```python
from build123d import *

# Parameters (mm, degrees)
SKETCH1_W                       = 165.076666628
SKETCH1_H                       = 208.28
BOSS_EXTRUDE1_DEPTH             = 89.481016872
SKETCH3_W                       = 161.266666628
SKETCH3_H                       = 208.28
CUT_EXTRUDE1_DEPTH              = 87.576016872
F_6_CLEARANCE_HOLE1_AT_2_COUNT  = 2
F_6_CLEARANCE_HOLE1_AT_2_PITCH  = 70.431016872
F_6_CLEARANCE_HOLE1_AT_3_COUNT  = 2
F_6_CLEARANCE_HOLE1_AT_3_PITCH  = 201.912161688
F_6_CLEARANCE_HOLE1_AT_4_COUNT  = 2
F_6_CLEARANCE_HOLE1_AT_4_PITCH  = 189.23
F_6_CLEARANCE_HOLE2_D           = 4.3053
F_6_CLEARANCE_HOLE2_DEPTH       = 6.858
F_6_CLEARANCE_HOLE2_CSINK_D     = 6.6548
F_6_CLEARANCE_HOLE2_CSINK_ANGLE = 90
F_6_CLEARANCE_HOLE2_TIP         = 1.293442612
CUT_EXTRUDE2_REACH              = 162.202
SKETCH8_R                       = 45.72
CUT_EXTRUDE3_REACH              = 162.202
SKETCH9_R                       = 6
SKETCH9_W                       = 101.6
SKETCH9_H                       = 25.4
CUT_EXTRUDE4_DEPTH              = 0.9525
CUT_EXTRUDE6_REACH              = 162.202
SKETCH13_R                      = 6.35
CUT_EXTRUDE7_DEPTH              = 1
CHAMFER1_SIZE                   = 1


# Read off the part's stored shape, not the designer's step: M2 Clearance Hole1
with BuildPart() as part:
    # Sketch1 → Boss-Extrude1 (new body)
    with BuildSketch(Plane(origin=(0, 0, 0), x_dir=(0, 0, -1), z_dir=(1, 0, 0))):
        Rectangle(SKETCH1_W, SKETCH1_H)
    extrude(amount=BOSS_EXTRUDE1_DEPTH)

    # Sketch3 → Cut-Extrude1 (cut)
    with BuildSketch(Plane.ZY):
        Rectangle(SKETCH3_W, SKETCH3_H)
    extrude(amount=-CUT_EXTRUDE1_DEPTH, mode=Mode.SUBTRACT)

    # Sketch5 → #6 Clearance Hole1 (revolve, cut)
    with BuildSketch(Plane(origin=(9.525, -94.615, -82.538333314), x_dir=(0, 1, 0), z_dir=(1, 0, 0))):
        Polygon((0, 0), (0, 1.905), (2.15265, 1.905), (2.15265, 1.17475), (3.3274, 0), align=None)
    f_6_clearance_hole1 = revolve(axis=Axis((9.525, -94.615, -88.888333314), (0, 0, 1)), mode=Mode.SUBTRACT)

    # #6 Clearance Hole1 at 2: #6 Clearance Hole1 ×2
    with Locations(*[(i * F_6_CLEARANCE_HOLE1_AT_2_PITCH, 0, 0) for i in range(1, F_6_CLEARANCE_HOLE1_AT_2_COUNT)]):
        add(f_6_clearance_hole1, mode=Mode.SUBTRACT)

    # #6 Clearance Hole1 at 3: #6 Clearance Hole1 ×2
    with Locations(*[Vector(0.34882008237197215, 0.9371897087217778, 0) * (i * F_6_CLEARANCE_HOLE1_AT_3_PITCH) for i in range(1, F_6_CLEARANCE_HOLE1_AT_3_COUNT)]):
        add(f_6_clearance_hole1, mode=Mode.SUBTRACT)

    # #6 Clearance Hole1 at 4: #6 Clearance Hole1 ×2
    with Locations(*[(0, i * F_6_CLEARANCE_HOLE1_AT_4_PITCH, 0) for i in range(1, F_6_CLEARANCE_HOLE1_AT_4_COUNT)]):
        add(f_6_clearance_hole1, mode=Mode.SUBTRACT)

    # #6 Clearance Hole2
    with Locations(Plane.XY.offset(82.538333314)):
        with Locations((9.525, 94.615), (79.956016872, 94.615), (79.956016872, -94.615), (9.525, -94.615)):
            CounterSinkHole(F_6_CLEARANCE_HOLE2_D / 2, F_6_CLEARANCE_HOLE2_CSINK_D / 2, depth=F_6_CLEARANCE_HOLE2_DEPTH, counter_sink_angle=F_6_CLEARANCE_HOLE2_CSINK_ANGLE)
            with Locations((0, 0, -(F_6_CLEARANCE_HOLE2_DEPTH + F_6_CLEARANCE_HOLE2_TIP / 2))):  # 118° drill point
                Cone(0, F_6_CLEARANCE_HOLE2_D / 2, F_6_CLEARANCE_HOLE2_TIP, mode=Mode.SUBTRACT)

    # Sketch8 → Cut-Extrude2 (cut, up to next)
    with BuildSketch(Plane(origin=(89.481016872, 0, 0), x_dir=(0, 0, -1), z_dir=(1, 0, 0)), mode=Mode.PRIVATE) as cut_extrude2_sk1:
        with Locations((15.193333225, 51.676666667)):
            Circle(SKETCH8_R)
    cut_extrude2_tool1 = extrude(cut_extrude2_sk1.sketch, amount=-CUT_EXTRUDE2_REACH, mode=Mode.PRIVATE) & part.part
    add(cut_extrude2_tool1.solids().sort_by_distance((89.481017, 51.676667, -15.193333))[0], mode=Mode.SUBTRACT)

    # Sketch9 → Cut-Extrude3 (cut, up to next)
    with BuildSketch(Plane(origin=(89.481016872, 0, 0), x_dir=(0, 0, -1), z_dir=(1, 0, 0)), mode=Mode.PRIVATE) as cut_extrude3_sk1:
        with Locations((55.233333314, -52.07)):
            Circle(SKETCH9_R)
    cut_extrude3_tool1 = extrude(cut_extrude3_sk1.sketch, amount=-CUT_EXTRUDE3_REACH, mode=Mode.PRIVATE) & part.part
    # Sketch9 → Cut-Extrude3 (cut, up to next)
    with BuildSketch(Plane(origin=(89.481016872, 0, 0), x_dir=(0, 0, -1), z_dir=(1, 0, 0)), mode=Mode.PRIVATE) as cut_extrude3_sk2:
        with Locations((-11.418333314, -33.02)):
            Rectangle(SKETCH9_W, SKETCH9_H)
    cut_extrude3_tool2 = extrude(cut_extrude3_sk2.sketch, amount=-CUT_EXTRUDE3_REACH, mode=Mode.PRIVATE) & part.part
    # Sketch9 → Cut-Extrude3 (cut, up to next)
    with BuildSketch(Plane(origin=(89.481016872, 0, 0), x_dir=(0, 0, -1), z_dir=(1, 0, 0)), mode=Mode.PRIVATE) as cut_extrude3_sk3:
        with Locations((-11.418333314, -71.12)):
            Rectangle(SKETCH9_W, SKETCH9_H)
    cut_extrude3_tool3 = extrude(cut_extrude3_sk3.sketch, amount=-CUT_EXTRUDE3_REACH, mode=Mode.PRIVATE) & part.part
    add(cut_extrude3_tool1.solids().sort_by_distance((89.481017, -52.07, -55.233333))[0], mode=Mode.SUBTRACT)
    add(cut_extrude3_tool2.solids().sort_by_distance((89.481017, -33.02, 11.418333))[0], mode=Mode.SUBTRACT)
    add(cut_extrude3_tool3.solids().sort_by_distance((89.481017, -71.12, 11.418333))[0], mode=Mode.SUBTRACT)

    # M2 Clearance Hole1 outline → M2 Clearance Hole1 (revolve, cut)
    with BuildSketch(Plane(origin=(0, -33.02, 65.393333314), x_dir=(0, 1, 0), z_dir=(0, 0, -1))):
        Polygon((0, 87.576016872), (1.3, 87.576016872), (1.3, 88.881016872), (1.9, 89.481016872), (0, 89.481016872), align=None)
    revolve(axis=Axis((0, -33.02, 65.393333314), (1, 0, 0)), mode=Mode.SUBTRACT)

    # M2 Clearance Hole1 2 outline → M2 Clearance Hole1 2 (revolve, cut)
    with BuildSketch(Plane(origin=(0, -33.02, -42.556666686), x_dir=(0, 1, 0), z_dir=(0, 0, -1))):
        Polygon((0, 87.576016872), (1.3, 87.576016872), (1.3, 88.881016872), (1.9, 89.481016872), (0, 89.481016872), align=None)
    revolve(axis=Axis((0, -33.02, -42.556666686), (1, 0, 0)), mode=Mode.SUBTRACT)

    # M2 Clearance Hole1 3 outline → M2 Clearance Hole1 3 (revolve, cut)
    with BuildSketch(Plane(origin=(0, -71.12, -42.556666686), x_dir=(0, 1, 0), z_dir=(0, 0, -1))):
        Polygon((0, 87.576016872), (1.3, 87.576016872), (1.3, 88.881016872), (1.9, 89.481016872), (0, 89.481016872), align=None)
    revolve(axis=Axis((0, -71.12, -42.556666686), (1, 0, 0)), mode=Mode.SUBTRACT)

    # M2 Clearance Hole1 4 outline → M2 Clearance Hole1 4 (revolve, cut)
    with BuildSketch(Plane(origin=(0, -71.12, 65.393333314), x_dir=(0, 1, 0), z_dir=(0, 0, -1))):
        Polygon((0, 87.576016872), (1.3, 87.576016872), (1.3, 88.881016872), (1.9, 89.481016872), (0, 89.481016872), align=None)
    revolve(axis=Axis((0, -71.12, 65.393333314), (1, 0, 0)), mode=Mode.SUBTRACT)

    # Sketch12 → Cut-Extrude4 (cut)
    with BuildSketch(Plane.ZY.offset(-87.576016872)):
        with BuildLine():
            Line((-39.381666686, -17.78), (62.218333314, -17.78))
            Line((62.218333314, -17.78), (66.304587615, -24.952694807))
            ThreePointArc((66.304587615, -24.952694807), (68.441333314, -33.02), (66.304587615, -41.087305193))
            Line((66.304587615, -41.087305193), (62.218333314, -48.26))
            Line((62.218333314, -48.26), (-39.381666686, -48.26))
            Line((-39.381666686, -48.26), (-43.467920986, -41.087305193))
            ThreePointArc((-43.467920986, -41.087305193), (-45.604666686, -33.02), (-43.467920986, -24.952694807))
            Line((-43.467920986, -24.952694807), (-39.381666686, -17.78))
        make_face()
        with BuildLine():
            Line((-43.467920986, -79.187305193), (-39.381666686, -86.36))
            Line((-39.381666686, -86.36), (62.218333314, -86.36))
            Line((62.218333314, -86.36), (66.304587615, -79.187305193))
            ThreePointArc((66.304587615, -79.187305193), (68.441333314, -71.12), (66.304587615, -63.052694807))
            Line((66.304587615, -63.052694807), (62.218333314, -55.88))
            Line((62.218333314, -55.88), (-39.381666686, -55.88))
            Line((-39.381666686, -55.88), (-43.467920986, -63.052694807))
            ThreePointArc((-43.467920986, -63.052694807), (-45.604666686, -71.12), (-43.467920986, -79.187305193))
        make_face()
    extrude(amount=-CUT_EXTRUDE4_DEPTH, mode=Mode.SUBTRACT)

    # Lettering Outline → Cut-Extrude6 (cut, up to next)
    with BuildSketch(Plane(origin=(89.481016872, 0, 0), x_dir=(0, 0, -1), z_dir=(1, 0, 0)), mode=Mode.PRIVATE) as cut_extrude6_sk1:
        Polygon((-62.218333314, 78.77), (-62.218333314, 75.383333333), (-52.058333314, 75.383333333), (-52.058333314, 71.996666667), (-62.218333314, 71.996666667), (-62.218333314, 61.836666667), (-55.444999981, 61.836666667), (-55.444999981, 68.61), (-48.671666648, 61.836666667), (-45.284999981, 61.836666667), (-45.284999981, 65.223333333), (-48.671666648, 68.61), (-45.284999981, 68.61), (-45.284999981, 78.77), align=None)
    cut_extrude6_tool1 = extrude(cut_extrude6_sk1.sketch, amount=-CUT_EXTRUDE6_REACH, mode=Mode.PRIVATE) & part.part
    # Lettering Outline → Cut-Extrude6 (cut, up to next)
    with BuildSketch(Plane(origin=(89.481016872, 0, 0), x_dir=(0, 0, -1), z_dir=(1, 0, 0)), mode=Mode.PRIVATE) as cut_extrude6_sk2:
        Polygon((-62.218333314, 80.463333333), (-62.218333314, 90.623333333), (-52.058333314, 90.623333333), (-52.058333314, 94.01), (-62.218333314, 94.01), (-62.218333314, 97.396666667), (-45.284999981, 97.396666667), (-45.284999981, 80.463333333), (-52.058333314, 80.463333333), (-52.058333314, 87.236666667), (-55.444999981, 87.236666667), (-55.444999981, 80.463333333), align=None)
    cut_extrude6_tool2 = extrude(cut_extrude6_sk2.sketch, amount=-CUT_EXTRUDE6_REACH, mode=Mode.PRIVATE) & part.part
    # Lettering Outline → Cut-Extrude6 (cut, up to next)
    with BuildSketch(Plane(origin=(89.481016872, 0, 0), x_dir=(0, 0, -1), z_dir=(1, 0, 0)), mode=Mode.PRIVATE) as cut_extrude6_sk3:
        Polygon((-62.218333314, 24.583333333), (-62.218333314, 34.743333333), (-52.058333314, 34.743333333), (-52.058333314, 38.13), (-62.218333314, 38.13), (-62.218333314, 41.516666667), (-45.284999981, 41.516666667), (-45.284999981, 24.583333333), (-52.058333314, 24.583333333), (-52.058333314, 31.356666667), (-55.444999981, 31.356666667), (-55.444999981, 24.583333333), align=None)
    cut_extrude6_tool3 = extrude(cut_extrude6_sk3.sketch, amount=-CUT_EXTRUDE6_REACH, mode=Mode.PRIVATE) & part.part
    # Lettering Outline → Cut-Extrude6 (cut, up to next)
    with BuildSketch(Plane(origin=(89.481016872, 0, 0), x_dir=(0, 0, -1), z_dir=(1, 0, 0)), mode=Mode.PRIVATE) as cut_extrude6_sk4:
        Polygon((-62.218333314, 5.956666667), (-62.218333314, 22.89), (-55.444999981, 22.89), (-55.444999981, 19.503333333), (-52.058333314, 16.116666667), (-52.058333314, 22.89), (-45.284999981, 22.89), (-45.284999981, 5.956666667), (-52.058333314, 5.956666667), (-52.058333314, 9.343333333), (-55.444999981, 12.73), (-55.444999981, 5.956666667), align=None)
    cut_extrude6_tool4 = extrude(cut_extrude6_sk4.sketch, amount=-CUT_EXTRUDE6_REACH, mode=Mode.PRIVATE) & part.part
    # Lettering Outline → Cut-Extrude6 (cut, up to next)
    with BuildSketch(Plane(origin=(89.481016872, 0, 0), x_dir=(0, 0, -1), z_dir=(1, 0, 0)), mode=Mode.PRIVATE) as cut_extrude6_sk5:
        Polygon((-62.218333314, 43.21), (-58.831666648, 43.21), (-58.831666648, 49.983333333), (-55.444999981, 49.983333333), (-55.444999981, 43.21), (-52.058333314, 43.21), (-52.058333314, 49.983333333), (-48.671666648, 49.983333333), (-48.671666648, 43.21), (-45.284999981, 43.21), (-45.284999981, 60.143333333), (-52.058333314, 60.143333333), (-52.058333314, 56.756666667), (-55.444999981, 56.756666667), (-55.444999981, 60.143333333), (-62.218333314, 60.143333333), align=None)
    cut_extrude6_tool5 = extrude(cut_extrude6_sk5.sketch, amount=-CUT_EXTRUDE6_REACH, mode=Mode.PRIVATE) & part.part
    add(cut_extrude6_tool1.solids().sort_by_distance((89.481017, 70.491481, 53.476681))[0], mode=Mode.SUBTRACT)
    add(cut_extrude6_tool2.solids().sort_by_distance((89.481017, 88.93, 53.243667))[0], mode=Mode.SUBTRACT)
    add(cut_extrude6_tool3.solids().sort_by_distance((89.481017, 33.05, 53.243667))[0], mode=Mode.SUBTRACT)
    add(cut_extrude6_tool4.solids().sort_by_distance((89.481017, 14.423333, 53.751667))[0], mode=Mode.SUBTRACT)
    add(cut_extrude6_tool5.solids().sort_by_distance((89.481017, 52.354, 53.751667))[0], mode=Mode.SUBTRACT)

    # Sketch13 → Cut-Extrude7 (cut)
    with BuildSketch(Plane.XY.offset(-80.633333314)):
        with Locations((79.956016872, 94.615)):
            Circle(SKETCH13_R)
    extrude(amount=-CUT_EXTRUDE7_DEPTH, mode=Mode.SUBTRACT)

    # Chamfer1
    chamfer1_edges = [part.edges().sort_by_distance(p)[0] for p in [
        (73.606016872, 94.615, -80.633333314),
    ]]
    chamfer(chamfer1_edges, length=CHAMFER1_SIZE - 0.0001)  # a hair under: the kernel refuses the full size


solid = part.part
```
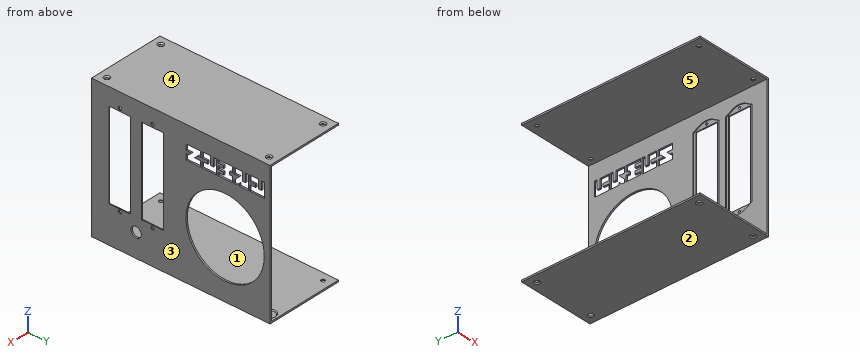
Design review of the part built by this model. Coordinates are the model's own, in mm. Face numbers are marked on the shaded views. A direction names the side the tool comes from. Coordinates: 2 decimals unless noted, no trailing zeros. Order: outer loops, then holes, each group sorted by start corner. A loop starts at its lowest first (then second) coordinate and runs counter-clockwise, first axis right, second up.
1) Wall thickness on line 1 along Z through (x, y) = (62.5, 23.5); line 2 along Z through (x, y) = (88.8, -33.02); line 3 along X through (y, z) = (80, -58): over which ranges is each line inside the solid? List them lowest first.
2) Take a section at C-C, the plane z = -35. Give the boundary of the cut face in (x, y).
3) Mouldability with a two-part tool opening along Z and no side actions: class the marked faces 1, 2 and 3 as +Z half, -Z half, draft (parallel to the pull), parting line (faces both ways), or undercut.
4) Take a section at B-B, the plane y = -52.07. Give the boundary of the cut face in (x, z), and give its area (3 significant figures).
5) For the marked faces 4 and 5, list the 3-axis set-ups (+Z, -Z, +X, -X, +Y, -Y) from which the entire face can be reached by the end or side of a thin tool; tool diameter is ignored.
6) Take a section at A-A, the plane x = 53.5. Give the boundary of the cut face in (y, z).
7) Take a section at D-D, the plane y = -2. Give the boundary of the cut face in (x, z).
8) Clearance check with flat-ended pins moving along their axes: pin 1 (5 mm diameter, centred on y = 34, z = 38.5, fed in from -X); pin 2 (15 mm diameter, centred on y = -40.5, z = 4.5, fed in from -X). State where each tip first meets the part, or that it passes through.
Returned:
1. line 1: z = -82.54 to -80.63, 80.63 to 82.54
1. line 2: z = -82.54 to -43.86, -41.26 to -39.38, 62.22 to 64.09, 66.69 to 82.54
1. line 3: x = 87.58 to 89.48
2. outline: (87.58, -104.14) - (89.48, -104.14) - (89.48, -83.82) - (88.53, -83.82) - (88.53, -86.36) - (87.58, -86.36) - close; (87.58, -55.88) - (88.53, -55.88) - (88.53, -58.42) - (89.48, -58.42) - (89.48, -45.72) - (88.53, -45.72) - (88.53, -48.26) - (87.58, -48.26) - close; (87.58, -17.78) - (88.53, -17.78) - (88.53, -20.32) - (89.48, -20.32) - (89.48, 10.47) - (87.58, 10.47) - close; (87.58, 92.88) - (89.48, 92.88) - (89.48, 104.14) - (87.58, 104.14) - close
3. face 1: undercut
3. face 2: -Z half
3. face 3: draft
4. outline: (0, -82.54) - (89.48, -82.54) - (89.48, -61.23) - (87.58, -61.23) - (87.58, -80.63) - (0, -80.63) - close; (0, 80.63) - (87.58, 80.63) - (87.58, -49.23) - (89.48, -49.23) - (89.48, 82.54) - (0, 82.54) - close
4. area: 625 mm2
5. face 4: +Z, +X, -X, +Y, -Y
5. face 5: -X, +Y, -Y
6. outline: (-104.14, -82.54) - (104.14, -82.54) - (104.14, -80.63) - (-104.14, -80.63) - close; (-104.14, 80.63) - (104.14, 80.63) - (104.14, 82.54) - (-104.14, 82.54) - close
7. outline: (0, -82.54) - (89.48, -82.54) - (89.48, 82.54) - (0, 82.54) - (0, 80.63) - (87.58, 80.63) - (87.58, -80.63) - (0, -80.63) - close
8. pin 1: stops at x = 87.58
8. pin 2: stops at x = 88.53
